Here's how the part is built. I have some questions about the finished solid (model axes, mm). Face numbers are marked on the shaded views. A direction names the side the tool comes from. Coordinates: 2 decimals unless noted, no trailing zeros. Loops run counter-clockwise (first coordinate to the right, second up) from the corner with the lowest first, then second, coordinate; pieces in that order, holes last. Notation, with made-up numbers: M 16,57.5 L 32,57.5 A30 ccw 32,91.5 Z; hole C 26.25,-27 d4. An arc over 180 degrees is marked long. Use CSV: the item, a comma, the result in double quotes. Start each with the question number.
Q1. If we mould it in two halves opening along X, with no side actions, what happens to the marked faces 1, 2, 3 and 4? For each: +X half, -X half, draft (parallel to the pull), parting line (faces both ways), or undercut.
Q2. If we section it at A-A (x = 30): Please give me the cut outline in (y, z), and give its area (3 significant figures).
Q3. Please list where these lines run through material, in increasing order: probe 1 along Y at (x, z) = (30, 10); probe 2 along Z at (x, y) = (-30, -2); probe 3 along Z at (x, y) = (-22.5, -0.5). Write a range as [from, to].
Q4. If we section it at B-B (z = 11): Please give me the cut outline in (x, y), and give its area (3 significant figures).
Q5. If we section it at C-C (y = -2): Please give me the cut outline in (x, z), and give its area (3 significant figures).
Q6. Which directions (+Z, -Z, +X, -X, +Y, -Y) give clear straight access to the entire face, cutting with the end or side of a thin tool? Please do the marked faces 5 and 6.
Q7. If we section it at D-D (x = 5): Please give me the cut outline in (y, z), and give its area (3 significant figures).
Q8. For pin 1 Ø1 at (y, z) = (7, 7) entering from +X; pin 2 Ø3.5 at (y, z) = (6, 7) entering from -X; pin 3 Ø3 at (y, z) = (-8, 14) entering from +X, each with a flat end and sliding along its axis, tell me the tip position at first contact or that it passes through.
from build123d import *

# Parameters (mm, degrees)
SKETCH_R          = 12.6
PAD_DEPTH         = 16
POCKET_DEPTH      = 20
POCKET_DEPTH_BACK = 20
POCKET001_DEPTH   = 16.001
SKETCH003_R       = 5.7
PAD001_DEPTH      = 11
SKETCH004_W       = 6
SKETCH004_H       = 22.8
POCKET002_DEPTH   = 5


with BuildPart() as part:
    # Sketch → Pad (new body)
    with BuildSketch(Plane.XY):
        with BuildLine():
            ThreePointArc((-30, 8.7), (-38.7, 0), (-30, -8.7))
            Line((-30, -8.7), (28.190735, -15.494727))
            ThreePointArc((28.190735, -15.494727), (45.6, 0), (28.190735, 15.494727))
            Line((-30, 8.7), (28.190735, 15.494727))
        make_face()
        with Locations((30, 0)):
            Circle(SKETCH_R, mode=Mode.SUBTRACT)
    extrude(amount=PAD_DEPTH)

    # Sketch001 → Pocket (cut, two sides)
    with BuildSketch(Plane.XZ) as pocket_sk:
        with BuildLine():
            Line((14.4, 0), (-21.3, 5))
            Line((-21.3, 5), (-25.212, 5))
            ThreePointArc((-25.212, 5), (-30, 13.792742), (-34.788, 5))
            Line((-34.788, 5), (-38.7, 5))
            Line((-38.7, 5), (-38.7, 0))
            Line((-38.7, 0), (14.4, 0))
        make_face()
    extrude(amount=-POCKET_DEPTH, mode=Mode.SUBTRACT)
    extrude(pocket_sk.sketch, amount=POCKET_DEPTH_BACK, mode=Mode.SUBTRACT)

    # Sketch002 (on Face9 of Pocket) → Pocket001 (cut, through all)
    with BuildSketch(Plane(origin=(0, 0, 0), x_dir=(1, 0, 0), z_dir=(0, 0, -1))):
        Polygon((30, 0), (62.76, 39.041848), (62.76, -39.041848), align=None)
    extrude(amount=-POCKET001_DEPTH, mode=Mode.SUBTRACT)

    # Sketch003 (on Face7 of Pocket) → Pad001 (join)
    with BuildSketch(Plane(origin=(0, 0, 5), x_dir=(1, 0, 0), z_dir=(0, 0, -1))):
        with BuildLine():
            ThreePointArc((-30, 8.7), (-38.7, 0), (-30, -8.7))
            Line((-21.3, -9.715868), (-30, -8.7))
            Line((-21.3, 9.715868), (-21.3, -9.715868))
            Line((-30, 8.7), (-21.3, 9.715868))
        make_face()
        with Locations((-30, 0)):
            Circle(SKETCH003_R, mode=Mode.SUBTRACT)
    extrude(amount=-PAD001_DEPTH)

    # Sketch004 (on Face9 of Pad001) → Pocket002 (cut)
    with BuildSketch(Plane(origin=(0, 0, 5), x_dir=(1, 0, 0), z_dir=(0, 0, -1))):
        with Locations((-30, 0)):
            Rectangle(SKETCH004_W, SKETCH004_H)
    extrude(amount=-POCKET002_DEPTH, mode=Mode.SUBTRACT)


solid = part.part
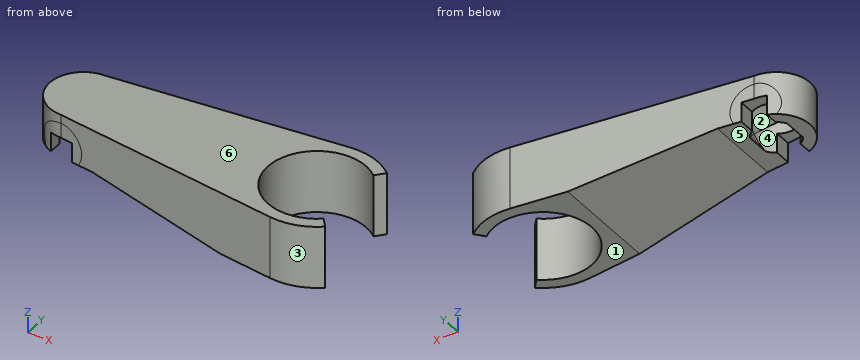
Results below:
1,face 1,"draft"
1,face 2,"undercut"
1,face 3,"parting line"
1,face 4,"undercut"
2,outline,"M -15.6,0 L -12.6,0 L -12.6,16 L -15.6,16 Z; M 12.6,0 L 15.6,0 L 15.6,16 L 12.6,16 Z"
2,area,"96.0 mm^2"
3,probe 1,"[-15.6, -12.6], [12.6, 15.6]"
3,probe 2,"[13.79, 16]"
3,probe 3,"[5, 16]"
4,outline,"M -30,-8.7 L 28.19,-15.49 A15.6 ccw 40.03,-11.95 L 38.1,-9.65 A12.6 cw long 38.1,9.65 L 40.03,11.95 A15.6 ccw 28.19,15.49 L -30,8.7 A8.7 ccw Z; hole M -34.9,-2.91 A5.7 ccw -25.1,-2.91 L -25.1,2.91 A5.7 ccw -34.9,2.91 Z"
4,area,"1,300 mm^2"
5,outline,"M -38.47,5 L -34.79,5 A5.7 cw -35.34,6.09 L -35.34,10.09 A5.7 cw -24.66,10.09 L -24.66,6.09 A5.7 cw -25.21,5 L -21.3,5 L 14.4,0 L 17.56,0 L 17.56,16 L -38.47,16 Z"
5,area,"639 mm^2"
6,face 5,"-Z, -X, +Y, -Y"
6,face 6,"+Z, +X, -X, +Y, -Y"
7,outline,"M -12.79,1.32 L 12.79,1.32 L 12.79,16 L -12.79,16 Z"
7,area,"376 mm^2"
8,pin 1,"x = 19.88"
8,pin 2,"x = -37.59"
8,pin 3,"x = 21.72"
